Drawing for the job (mm, zero at the part's lowest x, y, z). A direction names the side the tool comes from. Coordinates: 2 decimals unless noted, no trailing zeros. Order: outer loops, then holes, each group sorted by start corner. A loop starts at its lowest first (then second) coordinate and runs counter-clockwise, first axis right, second up. Notation, with made-up numbers: (41.25, 22) -> (80.25, 22) arc R34 ccw to (80.25, 54) -> close; hole circle Ø4 at (60.25, 58.5). An arc over 180 degrees is marked (long way). Write each question's results on one line, items separated by ' | '.
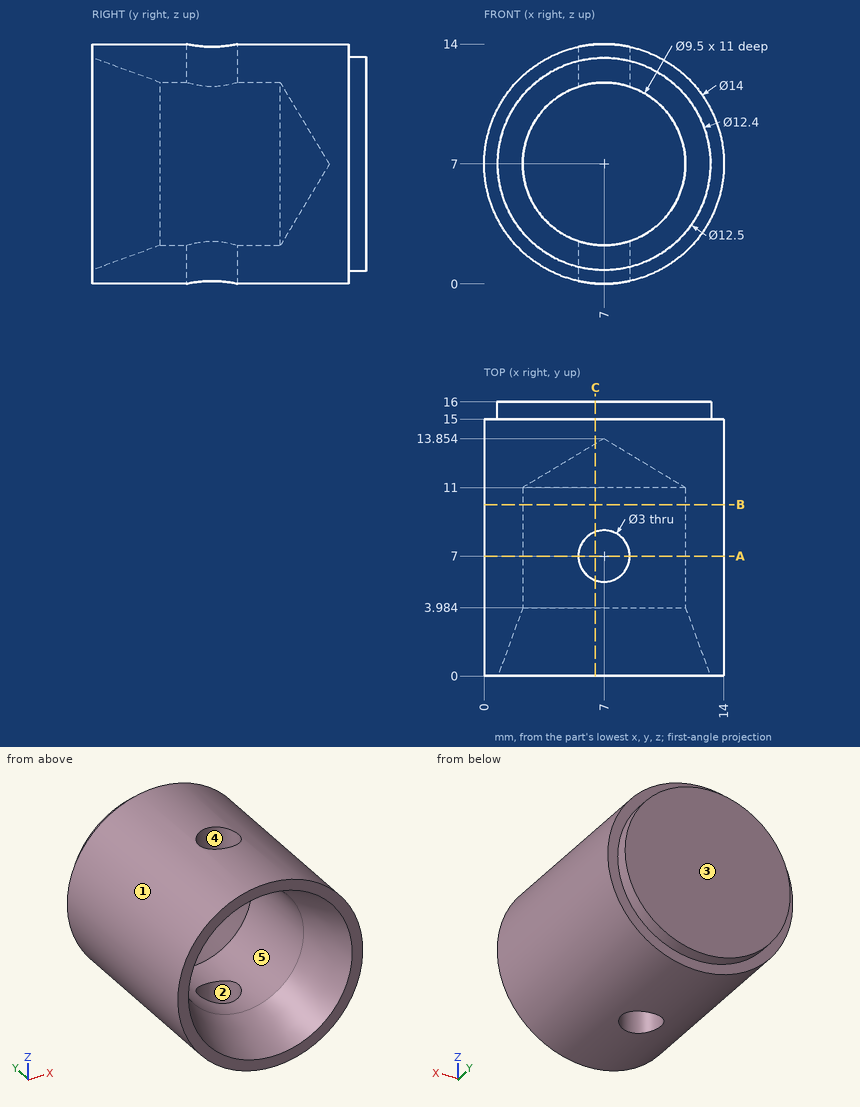
Item 1: Pull direction X, two halves, no side cores. Call the marked faces 1, 2 and 3: released by +X, released by -X, zero draft, split by the parting line, or undercut.
Answer:
face 1: split by the parting line | face 2: undercut | face 3: zero draft
Item 2: Drill centre lines: line 1 (X direction, y = 9, z = 7); line 2 (X direction, y = 14.5, z = 7.25); line 3 (X direction, y = 2.25, z = 6.5). Where is each one in solid material? Low to high. Write a range as from..to.
Answer:
line 1: x = 0..2.25, 11.75..14 | line 2: x = 0..14 | line 3: x = 0.02..1.64, 12.36..13.98
Item 3: Slice it at B-B, the plane y = 10. List the corners of the cut face in (x, z).
Answer:
outline: circle Ø14 at (7, 7); hole circle Ø9.5 at (7, 7)
Item 4: Tool access for the marked faces 4 and 5: list every direction of +Z, -Z, +X, -X, +Y, -Y with a clear straight run to the whole face (end or side of a thin tool).
Answer:
face 4: +Z, -Z | face 5: -Y
Item 5: Slice it at A-A, the plane y = 7. List the corners of the cut face in (x, z).
Answer:
outline: (5.5, 0.16) -> (5.5, 2.49) arc R4.75 cw to (5.5, 11.51) -> (5.5, 13.84) arc R7 ccw to start; (8.5, 0.16) arc R7 ccw to (8.5, 13.84) -> (8.5, 11.51) arc R4.75 cw to (8.5, 2.49) -> close
Item 6: Pin check, flat tips, straight feed: pin 1 (6 mm diameter, centred on y = 11.5, z = 7.5, fed in from -X); pin 2 (1 mm diameter, centred on y = 8, z = 4, fed in from +X); pin 3 (1.5 mm diameter, centred on x = 5, z = 5, fed in from -Y); pin 4 (1 mm diameter, centred on y = 12.5, z = 10, fed in from -X). Stop position of each tip, or through.
Answer:
pin 1: stops at x = 0 | pin 2: stops at x = 13.54 | pin 3: stops at y = 11.7 | pin 4: stops at x = 0.46
Item 7: Slice it at C-C, the plane x = 6.5. State how many separate pieces and enclosed holes the cut face has, and give its area (3 significant figures).
Answer:
separate pieces: 3 | enclosed holes: 0 | area: 86.4 mm^2
